Autodesk Inventor part; units mm, degrees
ref_plane "YZ Plane" through (0, 0, 0) normal (1, 0, 0) x (0, 1, 0)
ref_plane "XZ Plane" through (0, 0, 0) normal (0, 1, 0) x (-1, 0, 0)
ref_plane "XY Plane" through (0, 0, 0) normal (0, 0, 1) x (1, 0, 0)
sketch "Sketch1" plane through (0, 0, 0) normal (0, 1, 0) x (-1, 0, 0)
  circle A0 centre (0, 0) radius 3
  line L0 (-5, 10) -> (5, 10)
  line L1 (5, 10) -> (5, -10)
  line L2 (5, -10) -> (-5, -10)
  line L3 (-5, -10) -> (-5, 10)
  line L4 (-5, 10) -> (5, -10) construction
  line L5 (5, 10) -> (-5, -10) construction
  dimension "d0" = 6
  dimension "d1" = 10
  dimension "d2" = 20
extrude "Extrusion1" add sketch "Sketch1" along normal blind 6.36
properties part number "Brazo_eje"
CAD build for the part. Positions are in the model's coordinates, mm. Coordinates: 2 decimals unless noted, no trailing zeros. Order: outer loops, then holes, each group sorted by start corner. A loop starts at its lowest first (then second) coordinate and runs counter-clockwise, first axis right, second up. Notation, with made-up numbers: (-18.75, 81.25) - (-11.75, 81.25) arc R6 cw to (-11.75, 90.25) - close; hole circle Ø11 at (-14, 31). An arc over 180 degrees is marked (long way). Use a Markdown table: item, result. Add a question column.
(1) Pull direction Z, two halves, no side cores. Call faces 1 (the face through (2.3, 0, 2.4)), 2 (the face through (3, 3, 0)), 3 (the face through (0, 3, -10)): +Z half, -Z half, draft (parallel to the pull), parting line (faces both ways), or undercut.
(2) Drill centre lines: line 1 along Z through (x, y) = (0, 1.5); line 2 along Z through (x, y) = (-2, 4); line 3 along X through (y, z) = (5.75, 1.25). Where is each one in solid material? Low to high. Write a range as [from, to].
(3) Saw through at B-B (y = 1.5). Give the cut face in (x, z), then the cut area to 3 significant figures.
(4) Saw through at C-C (z = 0). Give the cut face in (x, y).
(5) Saw through at A-A (x = 0). Give the cut face in (y, z).
Solved:
| question | item | result |
|---|---|---|
| 1 | face 1 | draft |
| 1 | face 2 | undercut |
| 1 | face 3 | -Z half |
| 2 | line 1 | z = [-10, -3], [3, 10] |
| 2 | line 2 | z = [-10, -2.24], [2.24, 10] |
| 2 | line 3 | x = [-5, -2.73], [2.73, 5] |
| 3 | outline | (-5, -10) - (5, -10) - (5, 10) - (-5, 10) - close; hole circle Ø6 at (0, 0) |
| 3 | area | 172 mm² |
| 4 | outline | (-5, 0) - (-3, 0) - (-3, 6.36) - (-5, 6.36) - close; (3, 0) - (5, 0) - (5, 6.36) - (3, 6.36) - close |
| 5 | outline | (0, -10) - (6.36, -10) - (6.36, -3) - (0, -3) - close; (0, 3) - (6.36, 3) - (6.36, 10) - (0, 10) - close |
